from build123d import *

# Parameters (mm, degrees)
F0_W     = 25
F0_H     = 450
F1_DEPTH = 125
F2_DEPTH = 25
F3_START = 124.9
F0_W_2   = 400
F3_DEPTH = 25.1


with BuildPart() as f1:
    # F0 (on Top) → F1 (new body)
    with BuildSketch(Plane.XY):
        Polygon((-864.6446609407, -250), (-900, -250), (-1350, -700), (-1314.6446609407, -700), align=None)
        Polygon((-839.6446609407, -225), (-875, -225), (-900, -250), (-864.6446609407, -250), align=None)
        Polygon((-614.6446609407, 0), (-650, 0), (-875, -225), (-839.6446609407, -225), (-639.6446609407, -25), align=None)
        Polygon((0, -225), (-839.6446609407, -225), (-864.6446609407, -250), (-425, -250), (-400, -250), (0, -250), align=None)
        Polygon((0, 0), (-614.6446609407, 0), (-639.6446609407, -25), (0, -25), align=None)
        Polygon((614.6446609407, 0), (0, 0), (0, -25), (639.6446609407, -25), align=None)
        Polygon((839.6446609407, -225), (0, -225), (0, -250), (400, -250), (425, -250), (864.6446609407, -250), align=None)
        with Locations((412.5, -475)):
            Rectangle(F0_W, F0_H)
        with Locations((-412.5, -475)):
            Rectangle(F0_W, F0_H)
        Polygon((650, 0), (614.6446609407, 0), (639.6446609407, -25), (839.6446609407, -225), (875, -225), align=None)
        Polygon((900, -250), (864.6446609407, -250), (1314.6446609407, -700), (1350, -700), align=None)
        Polygon((875, -225), (839.6446609407, -225), (864.6446609407, -250), (900, -250), align=None)
    extrude(amount=F1_DEPTH)

    # F0 (on Top) → F2 (join)
    with BuildSketch(Plane.XY):
        Polygon((1314.6446609407, -700), (864.6446609407, -250), (425, -250), (425, -700), align=None)
        Polygon((839.6446609407, -225), (0, -225), (0, -250), (400, -250), (425, -250), (864.6446609407, -250), align=None)
        Polygon((875, -225), (839.6446609407, -225), (864.6446609407, -250), (900, -250), align=None)
        Polygon((900, -250), (864.6446609407, -250), (1314.6446609407, -700), (1350, -700), align=None)
        Polygon((650, 0), (614.6446609407, 0), (639.6446609407, -25), (839.6446609407, -225), (875, -225), align=None)
        Polygon((639.6446609407, -25), (0, -25), (0, -225), (839.6446609407, -225), align=None)
        with Locations((412.5, -475)):
            Rectangle(F0_W, F0_H)
        Polygon((614.6446609407, 0), (0, 0), (0, -25), (639.6446609407, -25), align=None)
        Polygon((0, 0), (-614.6446609407, 0), (-639.6446609407, -25), (0, -25), align=None)
        Polygon((0, -25), (-639.6446609407, -25), (-839.6446609407, -225), (0, -225), align=None)
        Polygon((0, -225), (-839.6446609407, -225), (-864.6446609407, -250), (-425, -250), (-400, -250), (0, -250), align=None)
        with Locations((-412.5, -475)):
            Rectangle(F0_W, F0_H)
        Polygon((-425, -250), (-864.6446609407, -250), (-1314.6446609407, -700), (-425, -700), align=None)
        Polygon((-614.6446609407, 0), (-650, 0), (-875, -225), (-839.6446609407, -225), (-639.6446609407, -25), align=None)
        Polygon((-839.6446609407, -225), (-875, -225), (-900, -250), (-864.6446609407, -250), align=None)
        Polygon((-864.6446609407, -250), (-900, -250), (-1350, -700), (-1314.6446609407, -700), align=None)
    extrude(amount=F2_DEPTH)

    # F0 (on Top) → F3 (join)
    with BuildSketch(Plane.XY.offset(F3_START)):
        Polygon((-614.6446609407, 0), (-650, 0), (-875, -225), (-839.6446609407, -225), (-639.6446609407, -25), align=None)
        Polygon((0, 0), (-614.6446609407, 0), (-639.6446609407, -25), (0, -25), align=None)
        Polygon((-839.6446609407, -225), (-875, -225), (-900, -250), (-864.6446609407, -250), align=None)
        Polygon((614.6446609407, 0), (0, 0), (0, -25), (639.6446609407, -25), align=None)
        Polygon((-864.6446609407, -250), (-900, -250), (-1350, -700), (-1314.6446609407, -700), align=None)
        Polygon((650, 0), (614.6446609407, 0), (639.6446609407, -25), (839.6446609407, -225), (875, -225), align=None)
        Polygon((-425, -250), (-864.6446609407, -250), (-1314.6446609407, -700), (-425, -700), align=None)
        with Locations((-412.5, -475)):
            Rectangle(F0_W, F0_H)
        with Locations((200, -475)):
            Rectangle(F0_W_2, F0_H)
        with Locations((-200, -475)):
            Rectangle(F0_W_2, F0_H)
        Polygon((875, -225), (839.6446609407, -225), (864.6446609407, -250), (900, -250), align=None)
        with Locations((412.5, -475)):
            Rectangle(F0_W, F0_H)
        Polygon((1314.6446609407, -700), (864.6446609407, -250), (425, -250), (425, -700), align=None)
        Polygon((900, -250), (864.6446609407, -250), (1314.6446609407, -700), (1350, -700), align=None)
        Polygon((639.6446609407, -25), (0, -25), (0, -225), (839.6446609407, -225), align=None)
        Polygon((0, -25), (-639.6446609407, -25), (-839.6446609407, -225), (0, -225), align=None)
        Polygon((839.6446609407, -225), (0, -225), (0, -250), (400, -250), (425, -250), (864.6446609407, -250), align=None)
        Polygon((0, -225), (-839.6446609407, -225), (-864.6446609407, -250), (-425, -250), (-400, -250), (0, -250), align=None)
    extrude(amount=F3_DEPTH)


solid = f1.part
Model file for the job. Use its own axes, mm. A direction names the side the tool comes from. Coordinates: 2 decimals unless noted, no trailing zeros. Order: outer loops, then holes, each group sorted by start corner. A loop starts at its lowest first (then second) coordinate and runs counter-clockwise, first axis right, second up. Notation, with made-up numbers: (-13, 24) -> (31, 24) arc R24 ccw to (31, 39) -> close; hole circle Ø2 at (62.5, 87.5). An arc over 180 degrees is marked (long way). Return JSON: item names as keys, results as strings. Group by question number.
Item 1: Pull direction X, two halves, no side cores. Call faces 5 (the flat face through (-19, -190, 0)), 6 (the flat face through (-777, -472, 124.9)), 7 (the flat face through (-995, -345, 74)): pulls with the +X half, pulls with the -X half, needs draft (parallel to the pull), parting line crosses it, or undercut.
Item 2: Saw through at C-C on y = -524.5. Write the cut outline in (x, z).
Item 3: Saw through at B-B on z = 77. Write the cut outline in (x, y), then the cut area to 3 significant figures.
Item 4: Wall check: line 1 along Z through (x, y) = (-446, -631.5); line 2 along Y through (x, z) = (440, 124.5); line 3 along X through (y, z) = (-653.5, 34.5). Give the ranges that are in metal, low to high. Write a range as [from, to].
Item 5: Tool access for faces 1 (the flat face through (765, -472, 25)), 2 (the flat face through (-19, -423, 150)), 3 (the flat face through (12, -225, 74)), 4 (the flat face through (400, -478, 62)): list every direction of +Z, -Z, +X, -X, +Y, -Y with a clear straight run to the whole face (end or side of a thin tool).
Item 6: Flat gauge pins, fed straight in: P1, Ø1, axis at x = -851.5, z = 17, coming from the +Y side; P2, Ø8, axis at x = -220.5, z = 62, coming from the -Y side; P3, Ø4, axis at x = -1059.5, z = 48, coming from the -Y side. Where does each tip first touch, or does it go through?
Item 7: Saw through at D-D on x = -974. Write the cut outline in (y, z).
Item 8: Saw through at A-A on x = -294.5. Write the cut outline in (y, z), then the cut area to 3 significant figures.
Values found:
{
 "1": {"face 5": "needs draft", "face 6": "undercut", "face 7": "pulls with the -X half"},
 "2": {"outline": "(-1174.5, 0) -> (-400, 0) -> (-400, 124.9) -> (400, 124.9) -> (400, 0) -> (1174.5, 0) -> (1174.5, 150) -> (-1174.5, 150) -> close; hole (-1139.14, 25) -> (-425, 25) -> (-425, 124.9) -> (-1139.14, 124.9) -> close; hole (425, 25) -> (1139.14, 25) -> (1139.14, 124.9) -> (425, 124.9) -> close"},
 "3": {"outline": "(-1350, -700) -> (-1314.64, -700) -> (-864.64, -250) -> (-425, -250) -> (-425, -700) -> (-400, -700) -> (-400, -250) -> (400, -250) -> (400, -700) -> (425, -700) -> (425, -250) -> (864.64, -250) -> (1314.64, -700) -> (1350, -700) -> (650, 0) -> (-650, 0) -> close; hole (-839.64, -225) -> (839.64, -225) -> (639.64, -25) -> (-639.64, -25) -> close", "area": "146,000 mm2"},
 "4": {"line 1": "z = [0, 25], [124.9, 150]", "line 2": "y = [-250, -225], [-25, 0]", "line 3": "x = [-1303.5, -1268.14], [-425, -400], [400, 425], [1268.14, 1303.5]"},
 "5": {"face 1": "-Y", "face 2": "+Z, +X, -X, +Y, -Y", "face 3": "none", "face 4": "-Z, -Y"},
 "6": {"P1": "stops at y = -201", "P2": "stops at y = -250", "P3": "stops at y = -446.86"},
 "7": {"outline": "(-700, 0) -> (-324, 0) -> (-324, 150) -> (-700, 150) -> (-700, 124.9) -> (-359.36, 124.9) -> (-359.36, 25) -> (-700, 25) -> close"},
 "8": {"outline": "(-700, 124.9) -> (-250, 124.9) -> (-250, 0) -> (0, 0) -> (0, 150) -> (-700, 150) -> close; hole (-225, 25) -> (-25, 25) -> (-25, 124.9) -> (-225, 124.9) -> close", "area": "28,800 mm2"}
}
